Verification items for the finished model (mm, model axes). Round coordinates to 2 decimals unless told otherwise and drop trailing zeros. Order: outer loops, then holes, each group sorted by start corner. A loop starts at its lowest first (then second) coordinate and runs counter-clockwise, first axis right, second up. Notation, with made-up numbers: M -39,41 L 18,41 A14 cw 18,60 Z; hole C 29.25,72 d4. An arc over 180 degrees is marked long. Write item = value, one per line. Start each with the question number.
from build123d import *

# Parameters (mm, degrees)
SKETCH1_W               = 38.1
SKETCH1_H               = 38.1
BOSS_EXTRUDE1_DEPTH     = 574.7363918
CUT_EXTRUDE1_DEPTH      = 578.256563461
CUT_EXTRUDE1_DEPTH_BACK = 578.256563461
CUT_EXTRUDE2_DEPTH      = 578.256563461
CUT_EXTRUDE2_DEPTH_BACK = 578.256563461


with BuildPart() as part:
    # Sketch1 → Boss-Extrude1 (new body)
    with BuildSketch(Plane(origin=(0, 0, 0), x_dir=(0, 0, -1), z_dir=(1, 0, 0))):
        with Locations((19.05, -19.05)):
            Rectangle(SKETCH1_W, SKETCH1_H)
    extrude(amount=BOSS_EXTRUDE1_DEPTH)

    # Sketch2 → Cut-Extrude1 (cut, two sides: drawn at the far end of the back side and taken through both)
    with BuildSketch(Plane.XY.offset(-CUT_EXTRUDE1_DEPTH_BACK)):
        Polygon((-1161.9957119, -38.1), (0, -38.1), (38.1, -38.1), (0, 0), (-821.655047595, 821.655047595), (-2982.499615844, 1677.042030058), (-3322.84028015, 817.286982464), align=None)
    extrude(amount=CUT_EXTRUDE1_DEPTH + CUT_EXTRUDE1_DEPTH_BACK, mode=Mode.SUBTRACT)

    # Sketch3 → Cut-Extrude2 (cut, two sides: drawn at the far end of the back side and taken through both)
    with BuildSketch(Plane.XY.offset(-CUT_EXTRUDE2_DEPTH_BACK)):
        Polygon((1736.7321037, -38.1), (574.7363918, -38.1), (536.6363918, -38.1), (574.7363918, 0), (1396.391439395, 821.655047595), (3557.236007644, 1677.042030058), (3897.57667195, 817.286982464), align=None)
    extrude(amount=CUT_EXTRUDE2_DEPTH + CUT_EXTRUDE2_DEPTH_BACK, mode=Mode.SUBTRACT)


solid = part.part
1) Scan lines: probe 1 along X at (y, z) = (-21, -31.5); probe 2 along X at (y, z) = (-15, -2.5); probe 3 along Y at (x, z) = (29, -3). Record each from-to range of solid material in increasing order.
2) Cross-section at A-A, the plane z = -13.5. Enter the section's corners in (x, y).
3) Gauge pin test, flat ends, axial feed: P1, Ø4, axis at y = -19, z = -11.5, coming from the -X side; P2, Ø1, axis at y = -10.5, z = -13, coming from the +X side; P3, Ø2, axis at y = -15, z = -21, coming from the -X side. Record the tip position at first contact, or that the pin passes through.
4) Cross-section at B-B, the plane y = -13. Enter the section's corners in (x, z).
Geometry results:
q1.probe_1 = 21 to 553.74
q1.probe_2 = 15 to 559.74
q1.probe_3 = -29 to 0
q2.outline = M 0,0 L 38.1,-38.1 L 536.64,-38.1 L 574.74,0 Z
q3.P1 = 17
q3.P2 = 564.74
q3.P3 = 14
q4.outline = M 13,-38.1 L 561.74,-38.1 L 561.74,0 L 13,0 Z
